Study the drawing (mm; zero at the part's minimum x, y, z) and answer. A direction names the side the tool comes from. Coordinates: 2 decimals unless noted, no trailing zeros. Loops run counter-clockwise (first coordinate to the right, second up) from the corner with the lowest first, then second, coordinate; pieces in that order, holes last.
Q1. Straight lines are drawn through the part: line 1 (Y direction, x = 158, z = 53.5) (1 decimal); line 2 (X direction, y = 100, z = 23.5). For each, find the intervals that lie inside material, in ascending order.
Q2. Section A-A (x = 131) is taken. Give the vertices of the cut face in (y, z) (1 decimal).
Q3. A flat-ended cylindrical pin translates along its axis: P1, Ø17.5, axis at x = 69, y = 117, coming from the +Z side. Find the tip coordinate at first contact, or state that the pin passes through.
Q4. Section C-C (y = 19) is taken. Give the vertices of the cut face in (x, z).
Q5. The mould has two halves that part along Y. Classify the marked faces 3, 4 and 5: pulls with the +Y half, pulls with the -Y half, needs draft (parallel to the pull), parting line crosses it, or undercut.
Q6. Which of the six approach directions +Z, -Z, +X, -X, +Y, -Y give full straight-line access (tool end or side, diameter ignored) to the marked faces 1 and 2?
Q7. Section D-D (z = 16.5) is taken. Give the vertices of the cut face in (x, y) (1 decimal), then the cut area to 3 significant figures.
Q8. Section B-B (z = 86) is taken. Give the vertices of the cut face in (x, y) (1 decimal).
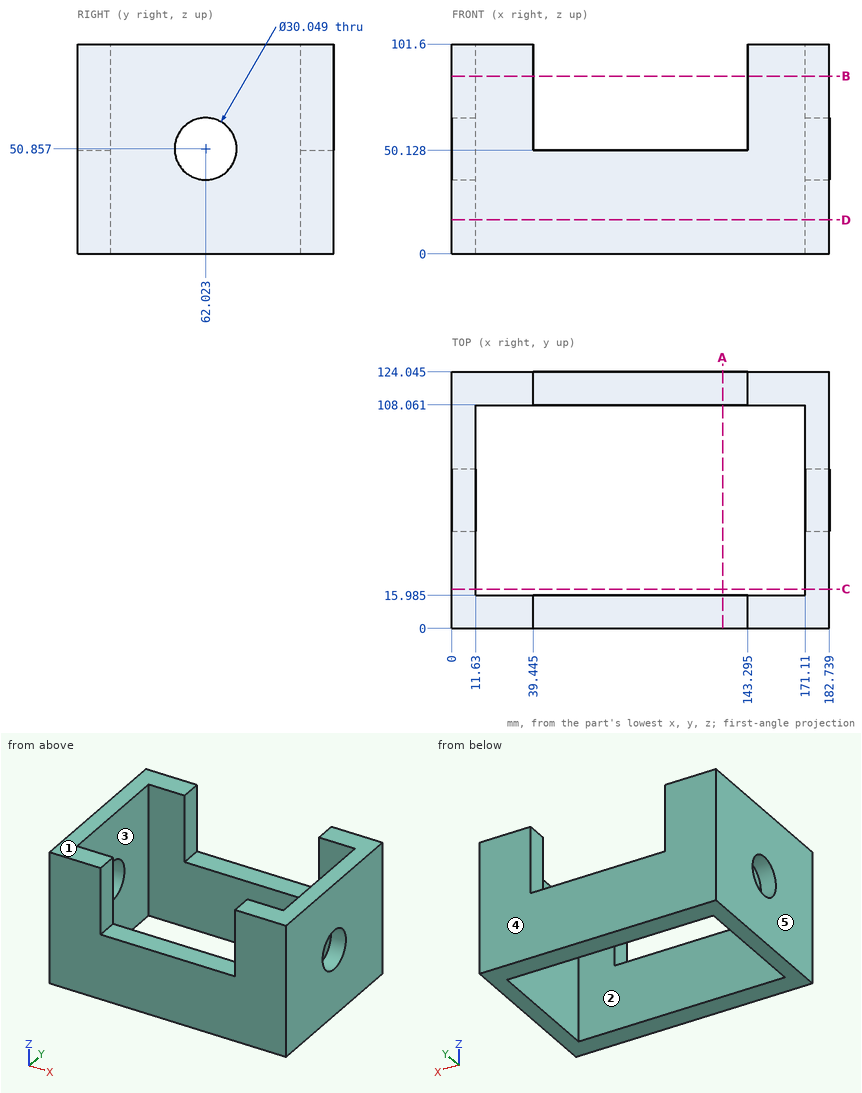
Numbers:
1. line 1: y = 0 to 16, 108.1 to 124
1. line 2: x = 0 to 11.63, 171.11 to 182.74
2. outline: (0, 0) - (16, 0) - (16, 50.1) - (0, 50.1) - close; (108.1, 0) - (124, 0) - (124, 50.1) - (108.1, 50.1) - close
3. P1: stops at z = 50.13
4. outline: (0, 0) - (11.63, 0) - (11.63, 101.6) - (0, 101.6) - close; (171.11, 0) - (182.74, 0) - (182.74, 101.6) - (171.11, 101.6) - close
5. face 3: undercut
5. face 4: pulls with the +Y half
5. face 5: needs draft
6. face 1: +Z, +X, -X, +Y, -Y
6. face 2: +Z, -Z
7. outline: (0, 0) - (182.7, 0) - (182.7, 124) - (0, 124) - close; hole (11.6, 16) - (171.1, 16) - (171.1, 108.1) - (11.6, 108.1) - close
7. area: 7,980 mm2
8. outline: (0, 0) - (39.4, 0) - (39.4, 16) - (11.6, 16) - (11.6, 108.1) - (39.4, 108.1) - (39.4, 124) - (0, 124) - close; (143.3, 0) - (182.7, 0) - (182.7, 124) - (143.3, 124) - (143.3, 108.1) - (171.1, 108.1) - (171.1, 16) - (143.3, 16) - close
